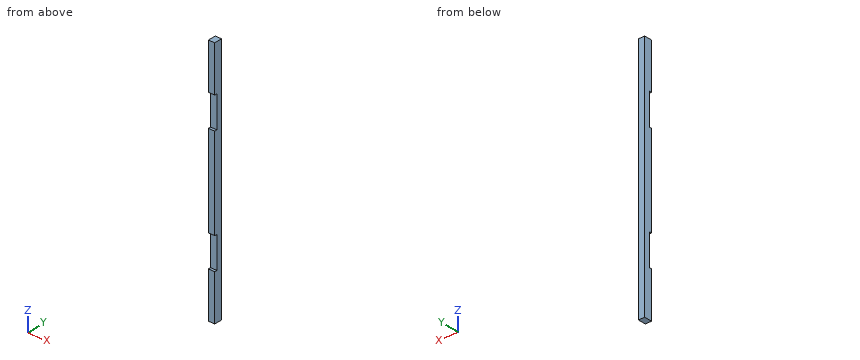
from build123d import *

# Parameters (mm, degrees)
EXTRUDE_1_OUTLINE_W = 25
EXTRUDE_1_OUTLINE_H = 780
EXTRUDE_1_DEPTH     = 20
SKETCH_2_W          = 100
SKETCH_2_H          = 8
CUT_EXTRUDE_1_DEPTH = 781.656774774


# Read off the part's stored shape, not the designer's step: Бобышка-Вытянуть1
with BuildPart() as part:
    # Бобышка-Вытянуть1 outline → Бобышка-Вытянуть1 (new body)
    with BuildSketch(Plane.YZ):
        with Locations((12.5, -390)):
            Rectangle(EXTRUDE_1_OUTLINE_W, EXTRUDE_1_OUTLINE_H)
    extrude(amount=EXTRUDE_1_DEPTH)

    # Эскиз2 → Вырез-Вытянуть1 (cut, through all)
    with BuildSketch(Plane(origin=(20, 0, 0), x_dir=(0, 0, -1), z_dir=(1, 0, 0))):
        with Locations((195, 4)):
            Rectangle(SKETCH_2_W, SKETCH_2_H)
        with Locations((585, 4)):
            Rectangle(SKETCH_2_W, SKETCH_2_H)
    extrude(amount=-CUT_EXTRUDE_1_DEPTH, mode=Mode.SUBTRACT)


solid = part.part
Can you work these out from the model? Positions are in its coordinate system, mm. Coordinates: 2 decimals unless noted, no trailing zeros. Order: outer loops, then holes, each group sorted by start corner. A loop starts at its lowest first (then second) coordinate and runs counter-clockwise, first axis right, second up. Notation, with made-up numbers: M 40.5,86.25 L 60.5,86.25 A14 cw 60.5,90.25 Z; hole C -2.5,65.25 d3. An arc over 180 degrees is marked long. Write item = value, one per line.
(1) I need wall thicknesses on line 1 along Z through (x, y) = (5.5, 4.25); line 2 along Y through (x, z) = (19, -588.5). Which ranges of each line are inside material? Lowest first, please. Write a range as [from, to].
Results are:
line_1 = [-780, -635], [-535, -245], [-145, 0]
line_2 = [8, 25]
(2) Suppose I cut it at B-B on x = 15.25. Please give me the cut outline in (y, z).
Results are:
outline = M 0,-780 L 25,-780 L 25,0 L 0,0 L 0,-145 L 8,-145 L 8,-245 L 0,-245 L 0,-535 L 8,-535 L 8,-635 L 0,-635 Z
(3) Suppose I cut it at A-A on y = 4.25. Please give me the cut outline in (x, z), plus the area to 3 significant figures.
Results are:
outline = M 0,-780 L 20,-780 L 20,-635 L 0,-635 Z; M 0,-535 L 20,-535 L 20,-245 L 0,-245 Z; M 0,-145 L 20,-145 L 20,0 L 0,0 Z
area = 11,600 mm2
(4) For pin 1 Ø2.5 at (x, y) = (5.5, 5.5) entering from +Z; pin 2 Ø10 at (x, z) = (12, -181.5) entering from -Y, each with a flat end and sliding along its axis, tell me the tip position at first contact or that it passes through.
Results are:
pin_1 = 0
pin_2 = 8
